Here's how the part is built. I have some questions about the finished solid (model axes, mm). A direction names the side the tool comes from. Round coordinates to 2 decimals unless told otherwise and drop trailing zeros. Loops run counter-clockwise (first coordinate to the right, second up) from the corner with the lowest first, then second, coordinate; pieces in that order, holes last. Notation, with made-up numbers: M 47.5,11.25 L 81.5,11.25 A6 cw 81.5,17.25 Z; hole C 49,81 d5. An arc over 180 degrees is marked long. Use a Markdown table: item, result.
```python
from build123d import *

# Parameters (mm, degrees)
F1_DEPTH = 19.05


with BuildPart() as f1:
    # F0 (on Top) → F1 (new body)
    with BuildSketch(Plane.XY):
        Polygon((-9.220245, 13.178808), (-44.145245, -28.803289), (-25.095245, -28.803289), (-9.220245, -12.35446), (6.654755, -28.803289), (25.704755, -28.803289), align=None)
        Polygon((-17.64437, -4.866622), (-8.822185, 4.268971), (0, -4.866622), align=None, mode=Mode.SUBTRACT)
    extrude(amount=F1_DEPTH)


solid = f1.part
```
Q1. I need wall thicknesses on line 1 (X direction, y = -2.5, z = 5.5); line 2 (X direction, y = -2, z = 1); line 3 (Y direction, x = 10.5, z = 15.25). Which ranges of each line are inside material? Lowest first, please. Write a range as from..to.
Return value:
| item | result |
|---|---|
| line 1 | x = -22.26..-15.36, -2.29..3.82 |
| line 2 | x = -21.85..-14.88, -2.77..3.41 |
| line 3 | y = -28.8..-10.53 |
Q2. For faces 1 (the flat face through (-1.394, -20.464, 9.392)), 2 (the flat face through (-10, -12, 0)), 3 (the flat face through (-13.295, -0.363, 9.392)), which set-ups out of +Z, -Z, +X, -X, +Y, -Y let a thin tool reach every point of the face, with its end or its side?
Return value:
| item | result |
|---|---|
| face 1 | +Z, -Z, -Y |
| face 2 | -Z, +X, -X, +Y, -Y |
| face 3 | +Z, -Z |
Q3. Imagine slicing it at B-B, the plane y = -20. Please give me the cut outline in (x, z), then the cut area to 3 significant figures.
Return value:
| item | result |
|---|---|
| outline | M -36.82,0 L -16.6,0 L -16.6,19.05 L -36.82,19.05 Z; M -1.84,0 L 18.38,0 L 18.38,19.05 L -1.84,19.05 Z |
| area | 770 mm^2 |
Q4. We'd pull the mould along Y, two halves only. Please class faces 4 (the flat face through (8.49, -8.11, 9.39)), 5 (the flat face through (-9, -4.867, 9)), 6 (the flat face through (-10, -12, 19.05)), 7 (the flat face through (16, -28.803, 9)): pulls with the +Y half, pulls with the -Y half, needs draft (parallel to the pull), parting line crosses it, or undercut.
Return value:
| item | result |
|---|---|
| face 4 | pulls with the +Y half |
| face 5 | undercut |
| face 6 | needs draft |
| face 7 | pulls with the -Y half |
Q5. Will these pins go through, and if not, where does the flat tip stop? P1, Ø8, axis at y = -10, z = 2.5, coming from the +X side; P2, Ø1, axis at x = -12.5, z = 9, coming from the +Y side; P3, Ø8, axis at y = -3, z = 16, coming from the +X side.
Return value:
| item | result |
|---|---|
| P1 | stops at x = 13.39 |
| P2 | stops at y = 9.84 |
| P3 | stops at x = 7.57 |
Q6. Imagine slicing it at A-A, the plane z = 11.5. Please give me the cut outline in (x, y).
Return value:
| item | result |
|---|---|
| outline | M -44.15,-28.8 L -25.1,-28.8 L -9.22,-12.35 L 6.65,-28.8 L 25.7,-28.8 L -9.22,13.18 Z; hole M -17.64,-4.87 L 0,-4.87 L -8.82,4.27 Z |
Q7. Imagine slicing it at D-D, the plane x = -29. Please give me the cut outline in (y, z).
Return value:
| item | result |
|---|---|
| outline | M -28.8,0 L -10.6,0 L -10.6,19.05 L -28.8,19.05 Z |
Q8. Imagine slicing it at C-C, the plane x = -7. Please give me the cut outline in (y, z), then the cut area to 3 significant figures.
Return value:
| item | result |
|---|---|
| outline | M -14.65,0 L -4.87,0 L -4.87,19.05 L -14.65,19.05 Z; M 2.38,0 L 10.51,0 L 10.51,19.05 L 2.38,19.05 Z |
| area | 341 mm^2 |
